The model under review builds one solid part; all positions refer to its coordinate system, in mm. A direction names the side the tool comes from. Give positions to 0.01 mm unless a question says otherwise; leave off trailing zeros. Order: outer loops, then holes, each group sorted by start corner. A loop starts at its lowest first (then second) coordinate and runs counter-clockwise, first axis right, second up.
Autodesk Inventor part; units mm, degrees
ref_plane "YZ Plane" through (0, 0, 0) normal (1, 0, 0) x (0, 1, 0)
ref_plane "XZ Plane" through (0, 0, 0) normal (0, 1, 0) x (-1, 0, 0)
ref_plane "XY Plane" through (0, 0, 0) normal (0, 0, 1) x (1, 0, 0)
sketch "Sketch1" plane through (0, 0, 0) normal (0, 1, 0) x (-1, 0, 0)
  line L0 (25, 50) -> (-25, 50)
  line L1 (-25, 50) -> (-25, -50)
  line L2 (-25, -50) -> (25, -50)
  line L3 (25, -50) -> (25, 50)
  line L4 (25, 50) -> (-25, -50) construction
  line L5 (-25, 50) -> (25, -50) construction
  circle A0 centre (-11, 38) radius 6.5
  circle A1 centre (-11, -38) radius 6.5
  point P0 (0, 0)
  dimension "d0" = 13
  dimension "d1" = 100
  dimension "d2" = 50
  dimension "d3" = 14
  dimension "d4" = 12
  dimension "d5" = 12
extrude "Extrusion1" add sketch "Sketch1" along normal blind 20
sketch "Sketch2" plane through (0, 20, 0) normal (0, 1, 0) x (1, 0, 0)
  circle A0 centre (11, -38) radius 6.5
  circle A1 centre (11, -38) radius 4
  circle A2 centre (11, 38) radius 6.5
  circle A3 centre (11, 38) radius 4
  point P0 (0, 0)
  dimension "d8" = 8
  dimension "d9" = 8
extrude "Extrusion2" add sketch "Sketch2" against normal blind 5
sketch "Sketch3" plane through (0, 0, 0) normal (0, -1, 0) x (1, 0, 0)
  circle A0 centre (-15, -30) radius 2.65
  circle A1 centre (-15, 30) radius 2.65
  line L0 (-25, -50) -> (-25, 50)
  line L1 (25, -50) -> (-25, -50)
  line L2 (-25, 50) -> (25, 50)
  point P0 (0, 0)
  dimension "d12" = 5.3
  dimension "d13" = 10
  dimension "d14" = 20
  dimension "d15" = 20
  dimension "d16" = 10
extrude "Extrusion3" cut sketch "Sketch3" against normal through all
fillet "Fillet1" radius 5 2 edges at (-25, 10, -50) (-25, 10, 50)
sketch "Sketch4" plane through (0, 20, 0) normal (0, 1, 0) x (1, 0, 0)
  circle A0 centre (-15, -30) radius 2.65
  line L0 (-19.734, -29.95) -> (-17.3237, -25.8752)
  line L1 (-17.3237, -25.8752) -> (-12.5897, -25.9252)
  line L2 (-12.5897, -25.9252) -> (-10.266, -30.05)
  line L3 (-10.266, -30.05) -> (-12.6763, -34.1248)
  line L4 (-12.6763, -34.1248) -> (-17.4103, -34.0748)
  line L5 (-17.4103, -34.0748) -> (-19.734, -29.95)
  circle A1 centre (-15, -30) radius 4.1
  circle A2 centre (-15, 30) radius 2.65
  line L6 (-19.7332, 30.1003) -> (-17.2797, 34.1492)
  line L7 (-17.2797, 34.1492) -> (-12.5465, 34.0489)
  line L8 (-12.5465, 34.0489) -> (-10.2668, 29.8997)
  line L9 (-10.2668, 29.8997) -> (-12.7203, 25.8508)
  line L10 (-12.7203, 25.8508) -> (-17.4535, 25.9511)
  line L11 (-17.4535, 25.9511) -> (-19.7332, 30.1003)
  circle A3 centre (-15, 30) radius 4.1
  point P0 (0, 0)
  dimension "d20" = 8.2
extrude "Extrusion4" [suppressed]
sketch "Sketch5" plane through (25, 0, 50) normal (1, 0, 0) x (0, 0, -1)
  line L0 (100, 0) -> (100, 20)
  line L1 (100, 20) -> (120, 20)
  line L2 (120, 20) -> (120, 0)
  line L3 (120, 0) -> (100, 0)
  line L4 (100, 0) -> (100, 20)
  circle A0 centre (110, 10) radius 2.75
  line L5 (0, 0) -> (0, 20)
  line L6 (0, 0) -> (-20, 0)
  line L7 (-20, 0) -> (-20, 20)
  line L8 (-20, 20) -> (0, 20)
  line L9 (0, 20) -> (0, 0)
  circle A1 centre (-10, 10) radius 2.75
  point P0 (50, 0)
  point P1 (0, 20)
  dimension "d23" = 20
  dimension "d24" = 5.5
  dimension "d27" = 20
  dimension "d28" = 20
  dimension "d29" = 20
  dimension "d30" = 5.5
extrude "Extrusion5" [suppressed]
chamfer "Chamfer1" [suppressed]
sketch "Sketch6" plane through (5, 0, 50) normal (-1, 0, 0) x (0, 0, 1)
  arc A0 (-110, 12.75) -> (-110, 7.25) centre (-110, 10) ccw
  circle A1 centre (-110, 10) radius 4.75
  circle A2 centre (10, 10) radius 2.75
  circle A3 centre (10, 10) radius 4.75
  point P0 (-50, 0)
  dimension "d34" = 9.5
extrude "Extrusion6" [suppressed]
fillet "Fillet2" [suppressed]
sketch "Sketch7" plane through (0, 20, 0) normal (0, 1, 0) x (1, 0, 0)
  circle A0 centre (-15, 30) radius 2.65
  circle A1 centre (-15, 30) radius 4.5
  circle A2 centre (-15, -30) radius 2.65
  circle A3 centre (-15, -30) radius 4.5
  point P0 (0, 0)
  dimension "d38" = 9
extrude "Extrusion7" cut sketch "Sketch7" against normal blind 5 contours A0 | A1 | A2 | A3
sketch "Sketch8" plane through (0, 0, 0) normal (0, -1, 0) x (1, 0, 0)
  circle A0 centre (11, 0) radius 4.1
  circle A1 centre (11, -38) radius 6.5
  line L0 (25, 50) -> (25, -50)
  line L1 (-20, 50) -> (25, 50)
  arc A2 (-20, 50) -> (-25, 45) centre (-20, 45) ccw
  line L2 (-25, -45) -> (-25, 45)
  arc A3 (-25, -45) -> (-20, -50) centre (-20, -45) ccw
  line L3 (25, -50) -> (-20, -50)
  circle A4 centre (-15, 30) radius 2.65
  circle A5 centre (-15, -30) radius 2.65
  circle A6 centre (11, 38) radius 6.5
  circle A7 centre (11, -38) radius 6.5
  point P0 (0, 0)
  dimension "d41" = 8.2
extrude "Extrusion8" cut sketch "Sketch8" against normal blind 10 contours A0
properties part number "Stationaryjaw"
Item 1: Draft analysis for pull direction Z (two halves, no side actions). For faces 3 (the flat face through (25, 10, 1)), 4 (the cylindrical face through (-23, 10, -49)), 5 (the flat face through (-13, 15, -28)), 6 (the flat face through (14, 15, -41)), state which applies: released by +Z, released by -Z, zero draft, split by the parting line, or undercut.
Values found:
face 3: zero draft
face 4: released by -Z
face 5: undercut
face 6: undercut
Item 2: Take a section at B-B (y = 18.25). Give the boundary of the cut face in (x, z), and give its area (3 significant figures).
Values found:
outline: (-25, -45) arc R5 ccw to (-20, -50) - (25, -50) - (25, 50) - (-20, 50) arc R5 ccw to (-25, 45) - close; hole circle Ø9 at (-15, -30); hole circle Ø9 at (-15, 30); hole circle Ø8 at (11, -38); hole circle Ø8 at (11, 38)
area: 4,760 mm2
Item 3: Take a section at D-D (y = 3.75). Give the boundary of the cut face in (x, z), and give its area (3 significant figures).
Values found:
outline: (-25, -45) arc R5 ccw to (-20, -50) - (25, -50) - (25, 50) - (-20, 50) arc R5 ccw to (-25, 45) - close; hole circle Ø5.3 at (-15, -30); hole circle Ø5.3 at (-15, 30); hole circle Ø13 at (11, -38); hole circle Ø13 at (11, 38); hole circle Ø8.2 at (11, 0)
area: 4,630 mm2
Item 4: For line 1 (Z direction, x = 11, y = 16.85); line 2 (Z direction, x = 11, y = 8.5); line 3 (Z direction, x = -15, y = 17.2), list the stretches that pass through material, from the lowest coordinate up.
Values found:
line 1: z = -50 to -42, -34 to 34, 42 to 50
line 2: z = -50 to -44.5, -31.5 to -4.1, 4.1 to 31.5, 44.5 to 50
line 3: z = -50 to -34.5, -25.5 to 25.5, 34.5 to 50
Item 5: Clearance check with flat-ended pins moving along their axes: pin 1 Ø5.5 at (x, z) = (-15, -30) entering from +Y; pin 2 Ø4 at (x, z) = (11, -1.5) entering from -Y; pin 3 Ø10.5 at (x, z) = (11, -38) entering from -Y. State where each tip first meets the part, or that it passes through.
Values found:
pin 1: stops at y = 15
pin 2: stops at y = 10
pin 3: stops at y = 15
Item 6: Take a section at C-C (x = -15). Give the boundary of the cut face in (y, z), and give its area (3 significant figures).
Values found:
outline: (0, -50) - (20, -50) - (20, -34.5) - (15, -34.5) - (15, -32.65) - (0, -32.65) - close; (0, -27.35) - (15, -27.35) - (15, -25.5) - (20, -25.5) - (20, 25.5) - (15, 25.5) - (15, 27.35) - (0, 27.35) - close; (0, 32.65) - (15, 32.65) - (15, 34.5) - (20, 34.5) - (20, 50) - (0, 50) - close
area: 1,750 mm2
Item 7: Take a section at A-A (z = 38). Give the boundary of the cut face in (x, y).
Values found:
outline: (-25, 0) - (4.5, 0) - (4.5, 15) - (7, 15) - (7, 20) - (-25, 20) - close; (15, 15) - (17.5, 15) - (17.5, 0) - (25, 0) - (25, 20) - (15, 20) - close
Item 8: For faces 1 (the cylindrical face through (-24, 10, 48)), 2 (the cylindrical face through (6.904, 4.93, 0.18)), list the 3-axis set-ups (+Z, -Z, +X, -X, +Y, -Y) from which the entire face can be reached by the end or side of a thin tool; tool diameter is ignored.
Values found:
face 1: +Z, -X, +Y, -Y
face 2: -Y
